from build123d import *

# Parameters (mm, degrees)
F1_DEPTH = 63.5
F2_DEPTH = 25.4
F3_DEPTH = 7.9375
F4_DEPTH = 25.4
F6_R     = 6.35


with BuildPart() as f1:
    # F0 (on Front) → F1 (new body, symmetric)
    with BuildSketch(Plane.XZ):
        Polygon((-41.275, 9.525), (-41.275, -9.525), (41.275, -9.525), (41.275, 9.525), (22.225, 9.525), align=None)
    extrude(amount=F1_DEPTH, both=True)

    # F0 (on Front) → F2 (join, symmetric)
    with BuildSketch(Plane.XZ):
        with BuildLine():
            Line((22.225, 9.525), (41.275, 9.525))
            Line((41.275, 9.525), (41.275, 27.0002))
            ThreePointArc((41.275, 27.0002), (45.92468, 38.22552), (57.15, 42.8752))
            Line((57.15, 42.8752), (60.325, 42.8752))
            Line((60.325, 42.8752), (60.325, 61.9252))
            Line((60.325, 61.9252), (57.15, 61.9252))
            add(Edge.make_bspline(
                [(54.548999, 61.828212), (55.417476, 61.872022), (56.284596, 61.904465), (57.15, 61.9252)],
                knots=[109.453159, 109.453159, 109.453159, 109.453159, 111.504536, 111.504536, 111.504536, 111.504536], degree=3))
            ThreePointArc((54.548999, 61.828212), (31.551215, 50.758521), (22.225, 27.0002))
            Line((22.225, 27.0002), (22.225, 9.525))
        make_face()
    extrude(amount=F2_DEPTH, both=True)

    # F0 (on Front) → F3 (join, symmetric)
    with BuildSketch(Plane.XZ):
        with BuildLine():
            add(Edge.make_bspline(
                [(-41.275, 9.525), (-41.989152, 24.791583), (8.210591, 59.490663), (54.548999, 61.828212)],
                knots=[0, 0, 0, 0, 109.453159, 109.453159, 109.453159, 109.453159], degree=3))
            Line((-41.275, 9.525), (22.225, 9.525))
            Line((22.225, 9.525), (22.225, 27.0002))
            ThreePointArc((22.225, 27.0002), (31.551215, 50.758521), (54.548999, 61.828212))
        make_face()
    extrude(amount=F3_DEPTH, both=True)

    # F0 (on Front) → F4 (join, symmetric)
    with BuildSketch(Plane.XZ):
        Polygon((71.658204, 61.9252), (60.325, 61.9252), (60.325, 42.8752), (71.658204, 42.8752), (85.725, 42.8752), (85.725, 61.9252), align=None)
    extrude(amount=F4_DEPTH, both=True)

    # F0 (on Front) → F5 (revolve)
    with BuildSketch(Plane.XZ):
        Polygon((111.125, 66.675), (85.725, 66.675), (85.725, 61.9252), (85.725, 42.8752), (85.725, 38.1), (111.125, 38.1), align=None)
    revolve(axis=Axis((85.725, 0, 52.3875), (0, 0, 1)))

    # F6
    f6_edges = [f1.edges().sort_by_distance(p)[0] for p in [
        (41.275, -63.5, 0),
        (-41.275, -63.5, 0),
        (41.275, 63.5, 0),
        (-41.275, 63.5, 0),
    ]]
    fillet(f6_edges, radius=F6_R)


solid = f1.part
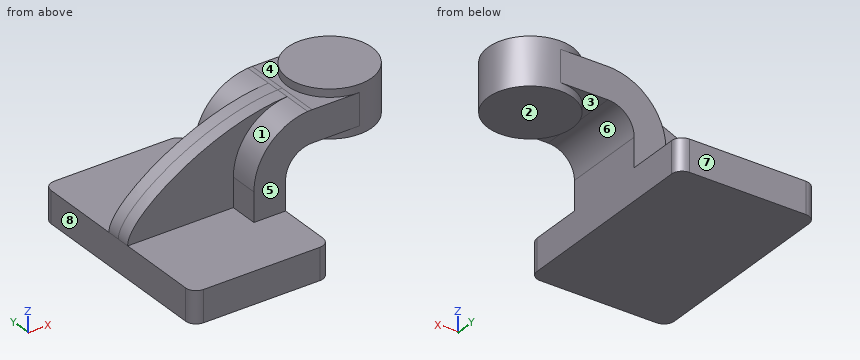
Source: CAD feature listing. Evaluate the final solid. Frame: model axes, mm. Face numbers are marked on the shaded views. A direction names the side the tool comes from. Give positions to 0.01 mm unless a question says otherwise; leave off trailing zeros. Write each loop counter-clockwise with the first axis right and the second up, starting at its lowest first coordinate (ties: lowest second). Pieces come first, ordered by that corner, then holes. Notation, with made-up numbers: (-15.75, 62.5) -> (28.25, 62.5) arc R12 cw to (28.25, 81.5) -> close; hole circle Ø11 at (82, -29.75). An arc over 180 degrees is marked (long way). Return JSON: item names as keys, results as strings. Group by question number.
1. Material intervals for line 1 (X direction, y = -15, z = 12) (3 decimals); line 2 (Y direction, x = 48.5, z = 42.5); line 3 (Z direction, x = 12.5, y = -17) (3 decimals), sorted ascending. Write a range as from..to.
2. Pin query (flat end, axial travel): pin 1 Ø1 at (x, y) = (50.5, 2) entering from +Z; pin 2 Ø1.5 at (y, z) = (2.5, 3) entering from -X (3 decimals); pin 3 Ø16.5 at (x, y) = (-10, 26.5) entering from +Z (3 decimals). Return the tip coordinate at first contact, or that it passes through.
3. Section D-D, the plane x = 88.5. Output: boundary loops of the cut face in (y, z) (3 decimals).
4. Section C-C, the plane x = 64. Output: boundary loops of the cut face in (y, z) (3 decimals).
5. Section A-A, the plane z = 3. Output: boundary loops of the cut face in (x, y) (3 decimals), then the cut area to 3 significant figures.
6. Mould query, pull axis X, two halves, no side actions, for the marked faces 6, 7 and 8. Classes: +X half, -X half, draft (parallel to the pull), parting line (faces both ways), or undercut.
7. Section B-B, the plane y = 45. Output: boundary loops of the cut face in (x, z) (3 decimals).
8. Access query for the marked faces 1, 2, 3, 4 and 5. Directions: +Z, -Z, +X, -X, +Y, -Y. A direction counts if a zero-diameter tool reaches every point of the face in a straight line with its end or side. Return the directions, or none.
Determined:
{
 "1": {"line 1": "x = 22.225..41.275", "line 2": "y = -25.4..25.4", "line 3": "z = -9.525..9.525"},
 "2": {"pin 1": "stops at z = 61.59", "pin 2": "stops at x = -41.275", "pin 3": "stops at z = 9.525"},
 "3": {"outline": "(-25.248, 38.1) -> (25.248, 38.1) -> (25.248, 66.675) -> (-25.248, 66.675) -> close"},
 "4": {"outline": "(-25.4, 42.875) -> (-13.16, 42.875) -> (-13.16, 38.1) -> (13.16, 38.1) -> (13.16, 42.875) -> (25.4, 42.875) -> (25.4, 61.925) -> (13.16, 61.925) -> (13.16, 66.675) -> (-13.16, 66.675) -> (-13.16, 61.925) -> (-25.4, 61.925) -> close"},
 "5": {"outline": "(-41.275, -57.15) arc R6.35 ccw to (-34.925, -63.5) -> (34.925, -63.5) arc R6.35 ccw to (41.275, -57.15) -> (41.275, 57.15) arc R6.35 ccw to (34.925, 63.5) -> (-34.925, 63.5) arc R6.35 ccw to (-41.275, 57.15) -> close", "area": "10,400 mm2"},
 "6": {"face 6": "undercut", "face 7": "draft", "face 8": "-X half"},
 "7": {"outline": "(-41.275, -9.525) -> (41.275, -9.525) -> (41.275, 9.525) -> (-41.275, 9.525) -> close"},
 "8": {"face 1": "+Z, -X, -Y", "face 2": "-Z, +X, +Y, -Y", "face 3": "-Z", "face 4": "+Z, -X", "face 5": "+Z, +X, -X, -Y"}
}
